Build history of the part. All positions in model axes, mm. Face numbers are marked on the shaded views. A direction names the side the tool comes from. Coordinates: 2 decimals unless noted, no trailing zeros. Write each loop counter-clockwise with the first axis right and the second up, starting at its lowest first coordinate (ties: lowest second). Pieces come first, ordered by that corner, then holes. Notation, with made-up numbers: (-29, 81.5) -> (5, 81.5) arc R9 ccw to (5, 86.5) -> close; hole circle Ø5 at (78.5, -9.5). An arc over 180 degrees is marked (long way). Write each question's results on one line, items separated by ' | '. Start each with the question number.
Q1. Saw through at C-C on y = 9.5. Give the cut face in (x, z), and give its area (3 significant figures).
Q2. Saw through at B-B on z = 9.25. Give the cut face in (x, y), and give its area (3 significant figures).
Q3. Saw through at D-D on z = 3.5. Count the separate pieces of the cut face and the enclosed holes in it, and give its area (3 significant figures).
Q4. Two-plate mould, pull along Y, no slides. Class the marked faces 3, 4 and 5: released by +Y, released by -Y, zero draft, split by the parting line, or undercut.
Q5. Saw through at A-A on x = 0. Give the cut face in (y, z) (3 decimals).
Q6. Drop flat-ended pins along their axis: pin 1 Ø4 at (x, z) = (15, 6.5) entering from +Y; pin 2 Ø3 at (x, z) = (5.5, 7.5) entering from +Y; pin 3 Ø1 at (y, z) = (8.5, 2) entering from -X. Give the stop position or say it passes through.
Q7. Tool access for the marked faces 1 and 2: list every direction of +Z, -Z, +X, -X, +Y, -Y with a clear straight run to the whole face (end or side of a thin tool).
Q8. Drill centre lines: line 1 (Z direction, x = -3, y = -7.5); line 2 (X direction, y = -2, z = 3.75); line 3 (X direction, y = -1, z = 1.75). Where is each one in solid material? Low to high.
from build123d import *

# Parameters (mm, degrees)
SKETCH1_R          = 24
EXTRUDE1_DEPTH     = 5
SKETCH2_R          = 5.5
EXTRUDE2_DEPTH     = 5
SKETCH3_R          = 2.5
CUT_EXTRUDE1_DEPTH = 11
SKETCH4_R          = 0.7
SKETCH4_R_2        = 0.66767911
CUT_EXTRUDE2_DEPTH = 6


with BuildPart() as part:
    # Sketch1 → Extrude1 (new body)
    with BuildSketch(Plane.XY):
        Circle(SKETCH1_R)
    extrude(amount=EXTRUDE1_DEPTH)

    # Sketch2 → Extrude2 (add)
    with BuildSketch(Plane.XY.offset(5)):
        Circle(SKETCH2_R)
    extrude(amount=EXTRUDE2_DEPTH)

    # Sketch3 → Cut-Extrude1 (cut, through all)
    with BuildSketch(Plane.XY.offset(10)):
        Circle(SKETCH3_R)
    extrude(amount=-CUT_EXTRUDE1_DEPTH, mode=Mode.SUBTRACT)

    # Sketch4 → Cut-Extrude2 (cut, through all)
    with BuildSketch(Plane.XY.offset(5)):
        with Locations((0, 20.73)):
            Circle(SKETCH4_R)
        with Locations((0, -20.73)):
            Circle(SKETCH4_R)
        with Locations((20.73, 0)):
            Circle(SKETCH4_R)
        with Locations((-20.73, 0)):
            Circle(SKETCH4_R)
        with Locations((-14.658, 14.658)):
            Circle(SKETCH4_R)
        with Locations((14.658, 14.658)):
            Circle(SKETCH4_R)
        with Locations((14.658, -14.658)):
            Circle(SKETCH4_R)
        with Locations((-14.658, -14.658)):
            Circle(SKETCH4_R)
        with Locations((19.152, 7.933)):
            Circle(SKETCH4_R)
        with Locations((7.933, 19.152)):
            Circle(SKETCH4_R)
        with Locations((19.152, -7.933)):
            Circle(SKETCH4_R)
        with Locations((7.933, -19.152)):
            Circle(SKETCH4_R)
        with Locations((-7.933, 19.152)):
            Circle(SKETCH4_R)
        with Locations((-19.152, 7.933)):
            Circle(SKETCH4_R)
        with Locations((-19.152, -7.933)):
            Circle(SKETCH4_R)
        with Locations((-7.933, -19.152)):
            Circle(SKETCH4_R)
        with Locations((20.331, 4.044)):
            Circle(SKETCH4_R)
        with Locations((20.331, -4.044)):
            Circle(SKETCH4_R)
        with Locations((4.044, -20.331)):
            Circle(SKETCH4_R)
        with Locations((-4.044, -20.331)):
            Circle(SKETCH4_R)
        with Locations((4.044, 20.331)):
            Circle(SKETCH4_R)
        with Locations((-4.044, 20.331)):
            Circle(SKETCH4_R_2)
        with Locations((-20.331, 4.044)):
            Circle(SKETCH4_R)
        with Locations((-20.331, -4.044)):
            Circle(SKETCH4_R)
        with Locations((17.236, 11.516)):
            Circle(SKETCH4_R)
        with Locations((11.516, 17.236)):
            Circle(SKETCH4_R)
        with Locations((17.236, -11.516)):
            Circle(SKETCH4_R)
        with Locations((11.516, -17.236)):
            Circle(SKETCH4_R)
        with Locations((-11.516, -17.236)):
            Circle(SKETCH4_R)
        with Locations((-17.236, -11.516)):
            Circle(SKETCH4_R)
        with Locations((-17.236, 11.516)):
            Circle(SKETCH4_R)
        with Locations((-11.516, 17.236)):
            Circle(SKETCH4_R)
        with Locations((0, 17.555)):
            Circle(SKETCH4_R)
        with Locations((17.555, 0)):
            Circle(SKETCH4_R)
        with Locations((0, -17.555)):
            Circle(SKETCH4_R)
        with Locations((-17.555, 0)):
            Circle(SKETCH4_R)
        with Locations((-12.413, 12.413)):
            Circle(SKETCH4_R)
        with Locations((12.413, 12.413)):
            Circle(SKETCH4_R)
        with Locations((12.413, -12.413)):
            Circle(SKETCH4_R)
        with Locations((-12.413, -12.413)):
            Circle(SKETCH4_R)
        with Locations((-16.218, 6.718)):
            Circle(SKETCH4_R)
        with Locations((16.218, 6.718)):
            Circle(SKETCH4_R)
        with Locations((16.218, -6.718)):
            Circle(SKETCH4_R)
        with Locations((-16.218, -6.718)):
            Circle(SKETCH4_R)
        with Locations((6.718, 16.218)):
            Circle(SKETCH4_R)
        with Locations((6.718, -16.218)):
            Circle(SKETCH4_R)
        with Locations((-6.718, -16.218)):
            Circle(SKETCH4_R)
        with Locations((-6.718, 16.218)):
            Circle(SKETCH4_R)
    extrude(amount=-CUT_EXTRUDE2_DEPTH, mode=Mode.SUBTRACT)


solid = part.part
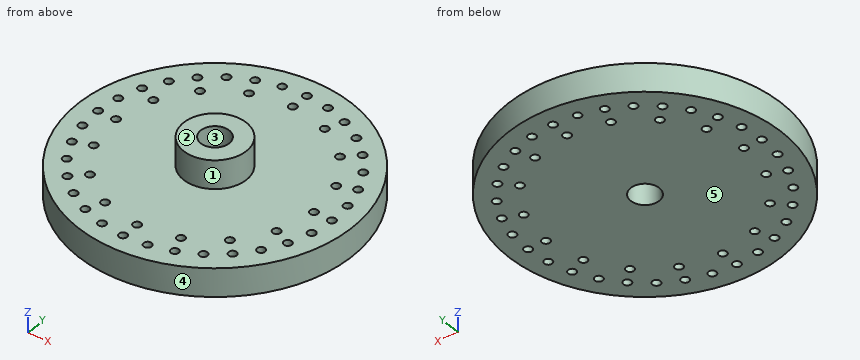
Returned:
1) outline: (-22.04, 0) -> (22.04, 0) -> (22.04, 5) -> (-22.04, 5) -> close | area: 220 mm2
2) outline: circle Ø11 at (0, 0); hole circle Ø5 at (0, 0) | area: 75.4 mm2
3) separate pieces: 1 | enclosed holes: 49 | area: 1,720 mm2
4) face 3: undercut | face 4: split by the parting line | face 5: zero draft
5) outline: (-24, 0) -> (-21.43, 0) -> (-21.43, 5) -> (-24, 5) -> close; (-20.03, 0) -> (-18.255, 0) -> (-18.255, 5) -> (-20.03, 5) -> close; (-16.855, 0) -> (-2.5, 0) -> (-2.5, 10) -> (-5.5, 10) -> (-5.5, 5) -> (-16.855, 5) -> close; (2.5, 0) -> (16.855, 0) -> (16.855, 5) -> (5.5, 5) -> (5.5, 10) -> (2.5, 10) -> close; (18.255, 0) -> (20.03, 0) -> (20.03, 5) -> (18.255, 5) -> close; (21.43, 0) -> (24, 0) -> (24, 5) -> (21.43, 5) -> close
6) pin 1: stops at y = 19.72 | pin 2: stops at y = 3.77 | pin 3: stops at x = -22.63
7) face 1: +Z | face 2: +Z, +X, -X, +Y, -Y
8) line 1: z = 0 to 5 | line 2: x = -23.92 to -1.5, 1.5 to 23.92 | line 3: x = -23.98 to -2.29, 2.29 to 23.98
